Can you work these out from the model? Positions are in its coordinate system, mm. Face numbers are marked on the shaded views. Give positions to 0.01 mm unless a question says otherwise; leave off trailing zeros. Loops run counter-clockwise (first coordinate to the right, second up) from the corner with the lowest first, then second, coordinate; pieces in that order, holes last. Notation, with made-up numbers: M 50,29.25 L 104,29.25 A26 cw 104,62.25 Z; hole C 41,54 d11. An arc over 180 degrees is marked long. Use CSV: the item, a comma, the result in double quotes.
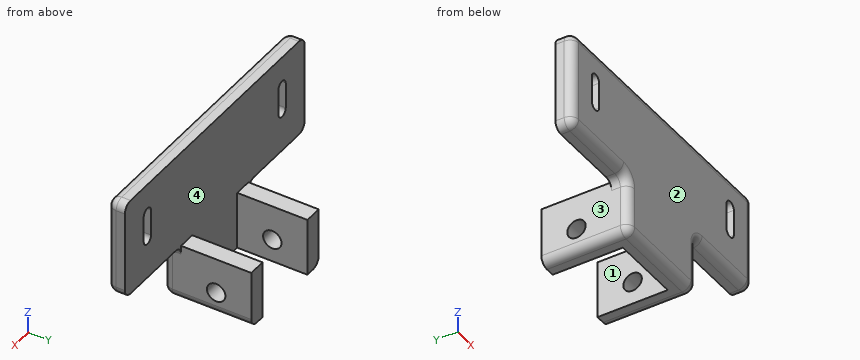
from build123d import *

# Parameters (mm, degrees)
BOSS_EXTRUDE1_START = 10
SKETCH1_W           = 16.5
SKETCH1_H           = 20
SKETCH1_R           = 2.625
BOSS_EXTRUDE1_DEPTH = 5
BOSS_EXTRUDE2_START = -10
SKETCH1_3_W         = 16.5
SKETCH1_3_H         = 20
SKETCH1_3_R         = 2.625
BOSS_EXTRUDE2_DEPTH = 5
BOSS_EXTRUDE3_START = -15
SKETCH1_4_W         = 16.5
SKETCH1_4_H         = 5
SKETCH1_4_W_2       = 28
BOSS_EXTRUDE3_DEPTH = 30
SKETCH2_W           = 25
SKETCH2_H           = 28
BOSS_EXTRUDE4_DEPTH = 5
FILLET1_R           = 2.5


with BuildPart() as part:
    # Sketch1 → Boss-Extrude1 (new body)
    with BuildSketch(Plane(origin=(0, 0, 0), x_dir=(0, 0, -1), z_dir=(1, 0, 0)).offset(BOSS_EXTRUDE1_START)):
        with Locations((-1.75, 0)):
            Rectangle(SKETCH1_W, SKETCH1_H)
        Circle(SKETCH1_R, mode=Mode.SUBTRACT)
    extrude(amount=BOSS_EXTRUDE1_DEPTH)



with BuildPart() as body_2:
    # Sketch1<3> → Boss-Extrude2 (new body)
    with BuildSketch(Plane(origin=(0, 0, 0), x_dir=(0, 0, -1), z_dir=(1, 0, 0)).offset(BOSS_EXTRUDE2_START)):
        with Locations((-1.75, 0)):
            Rectangle(SKETCH1_3_W, SKETCH1_3_H)
        Circle(SKETCH1_3_R, mode=Mode.SUBTRACT)
    extrude(amount=-BOSS_EXTRUDE2_DEPTH)


with BuildPart() as part_1:
    add(part.part)

    add(body_2.part)  # Boss-Extrude3 merges body 2
    # Sketch1<4> → Boss-Extrude3 (add)
    with BuildSketch(Plane(origin=(0, 0, 0), x_dir=(0, 0, -1), z_dir=(1, 0, 0)).offset(BOSS_EXTRUDE3_START)):
        with Locations((-1.75, -12.5)):
            Rectangle(SKETCH1_4_W, SKETCH1_4_H)
        with Locations((-24, -12.5)):
            Rectangle(SKETCH1_4_W_2, SKETCH1_4_H)
    extrude(amount=BOSS_EXTRUDE3_DEPTH)

    # Sketch2 → Boss-Extrude4 (add)
    with BuildSketch(Plane(origin=(0, -10, 0), x_dir=(1, 0, 0), z_dir=(0, 1, 0))):
        with Locations((-27.5, -24)):
            Rectangle(SKETCH2_W, SKETCH2_H)
        with BuildLine():
            Line((-31.625, -29.25), (-31.625, -21.75))
            ThreePointArc((-31.625, -21.75), (-30, -20.125), (-28.375, -21.75))
            Line((-28.375, -21.75), (-28.375, -29.25))
            ThreePointArc((-28.375, -29.25), (-30, -30.875), (-31.625, -29.25))
        make_face(mode=Mode.SUBTRACT)
        with Locations((27.5, -24)):
            Rectangle(SKETCH2_W, SKETCH2_H)
        with BuildLine():
            Line((31.625, -29.25), (31.625, -21.75))
            ThreePointArc((31.625, -21.75), (30, -20.125), (28.375, -21.75))
            Line((28.375, -21.75), (28.375, -29.25))
            ThreePointArc((28.375, -29.25), (30, -30.875), (31.625, -29.25))
        make_face(mode=Mode.SUBTRACT)
    extrude(amount=-BOSS_EXTRUDE4_DEPTH)

    # Fillet1
    fillet1_edges = [part_1.edges().sort_by_distance(p)[0] for p in [
        (0, -15, -6.5),
        (-15, -2.5, -6.5),
        (0, -15, 38),
        (-15, -15, 1.75),
        (15, -2.5, -6.5),
        (15, -15, 1.75),
        (-40, -12.5, 38),
        (-40, -12.5, 10),
        (-15, -12.5, 10),
        (-40, -15, 24),
        (-27.5, -15, 10),
        (27.5, -15, 10),
        (15, -12.5, 10),
        (40, -15, 24),
        (40, -12.5, 10),
        (40, -12.5, 38),
    ]]
    fillet(fillet1_edges, radius=FILLET1_R)


solid = part_1.part
Q1. I want a section at C-C, the plane z = 0. Please give me the cut outline in (x, y) (3 decimals), then the cut area to 3 significant figures.
Model answer:
outline,"M -15,-12.5 A2.5 ccw -12.5,-15 L 12.5,-15 A2.5 ccw 15,-12.5 L 15,-2.625 L 10,-2.625 L 10,-10 L -10,-10 L -10,-2.625 L -15,-2.625 Z; M -15,2.625 L -10,2.625 L -10,10 L -15,10 Z; M 10,2.625 L 15,2.625 L 15,10 L 10,10 Z"
area,"295 mm2"
Q2. I'm going to push flat-ended pins straight in: P1, Ø4, axis at y = 0, z = 0, coming from the +X side; P2, Ø1.5, axis at y = -13.5, z = 27, coming from the +X side; P3, Ø8.5, axis at y = 0, z = 0, coming from the +X side; P4, Ø0.8, axis at x = 24.5, y = -11.5, coming from the -Z side. Where does each tip first touch, or does it pass through?
Model answer:
P1,"through"
P2,"x = 39.99"
P3,"x = 15"
P4,"z = 10"
Q3. Please list where these lines run through material, in increasing order: L1, parallel to Y at x = -12, z = 0 (3 decimals); L2, parallel to X at y = 4.5, z = -0.5; L3, parallel to Y at x = 1.5, z = 18. Write a range as from..to.
Model answer:
L1,"-15..-2.625, 2.625..10"
L2,"-15..-10, 10..15"
L3,"-15..-10"
Q4. I want a section at D-D, the plane y = 5.75. Please give me the cut outline in (x, z).
Model answer:
outline,"M -15,-4 A2.5 ccw -12.5,-6.5 L -10,-6.5 L -10,10 L -15,10 Z; M 10,-6.5 L 12.5,-6.5 A2.5 ccw 15,-4 L 15,10 L 10,10 Z"
Q5. I want a section at B-B, the plane y = 0. Please give me the cut outline in (x, z) (3 decimals).
Model answer:
outline,"M -15,-4 A2.5 ccw -12.5,-6.5 L -10,-6.5 L -10,-2.625 L -15,-2.625 Z; M -15,2.625 L -10,2.625 L -10,10 L -15,10 Z; M 10,-6.5 L 12.5,-6.5 A2.5 ccw 15,-4 L 15,-2.625 L 10,-2.625 Z; M 10,2.625 L 15,2.625 L 15,10 L 10,10 Z"
Q6. I want a section at A-A, the plane x = 30. Please give me the cut outline in (y, z) (3 decimals), then the cut area to 3 significant figures.
Model answer:
outline,"M -15,12.5 A2.5 ccw -12.5,10 L -10,10 L -10,20.125 L -15,20.125 Z; M -15,30.875 L -10,30.875 L -10,38 L -12.5,38 A2.5 ccw -15,35.5 Z"
area,"83.6 mm2"
Q7. If we mould it in two halves opening along X, with no side actions, what happens to the marked faces 1, 2, 3 and 4? For each: released by +X, released by -X, zero draft, split by the parting line, or undercut.
Model answer:
face 1,"undercut"
face 2,"zero draft"
face 3,"released by -X"
face 4,"undercut"
